Could you check a few things on this model? Use its own coordinates, in mm. Face numbers are marked on the shaded views. Round coordinates to 2 decimals unless told otherwise and drop trailing zeros. Loops run counter-clockwise (first coordinate to the right, second up) from the corner with the lowest first, then second, coordinate; pieces in that order, holes last. Notation, with made-up numbers: (2, 16) -> (6, 16) arc R35 cw to (6, 50) -> close; hole circle Ø3 at (16.25, -34.5). An arc over 180 degrees is marked (long way). Write each question's results on one line, items separated by ' | '. Start each with the question number.
1) Imagine slicing it at B-B, the plane y = 6.25. List the corners of the cut face in (x, z) for me (3 decimals), plus the area to 3 significant figures.
2) For P1, Ø4, axis at x = 47.5, z = -9, coming from the +Y side; P2, Ø1.5, axis at x = 37, y = 4.5, coming from the -Z side, each with a flat end and sliding along its axis, tell me the tip position at first contact or that it passes through.
3) Imagine slicing it at A-A, the plane z = -19.05. List the corners of the cut face in (x, y) for me (3 decimals).
4) If I drill on probe 1 along X at (y, z) = (1.05, -19.05) (3 decimals); probe 2 along X at (y, z) = (7.25, -5.5); probe 3 along X at (y, z) = (1.25, -20.5), over which ranges is the centre line in solid material (lowest first)?
5) Imagine slicing it at C-C, the plane x = 97.79. List the corners of the cut face in (y, z) for me (3 decimals).
6) We'd pull the mould along X, two halves only. Please class the marked faces 1 and 2: pulls with the +X half, pulls with the -X half, needs draft (parallel to the pull), parting line crosses it, or undercut.
7) Imagine slicing it at D-D, the plane z = -7.5. List the corners of the cut face in (x, y) for me, plus the area to 3 significant figures.
from build123d import *

# Parameters (mm, degrees)
BASE_R                 = 1.905
BOSS_EXTRUDEBASE_DEPTH = 2.54
STANDOFFS_R            = 3.175
STANDOFFS_R_2          = 1.27
BOSS_EXTRUDE2_DEPTH    = 5.08


with BuildPart() as part:
    # Base → Boss-ExtrudeBase (new body)
    with BuildSketch(Plane(origin=(0, 0, 0), x_dir=(1, 0, 0), z_dir=(0, 1, 0))):
        with BuildLine():
            Line((2.54, 0), (99.06, 0))
            ThreePointArc((99.06, 0), (100.856051224, 0.743948776), (101.6, 2.54))
            Line((101.6, 2.54), (101.6, 35.56))
            ThreePointArc((101.6, 35.56), (100.856051224, 37.356051224), (99.06, 38.1))
            Line((99.06, 38.1), (2.54, 38.1))
            ThreePointArc((2.54, 38.1), (0.743948776, 37.356051224), (0, 35.56))
            Line((0, 35.56), (0, 2.54))
            ThreePointArc((0, 2.54), (0.743948776, 0.743948776), (2.54, 0))
        make_face()
        with Locations(Location((3.81, 19.05, 0), (0, 0, 270))):
            Circle(BASE_R, mode=Mode.SUBTRACT)
        with Locations(Location((97.79, 19.05, 0), (0, 0, 90))):
            Circle(BASE_R, mode=Mode.SUBTRACT)
    extrude(amount=BOSS_EXTRUDEBASE_DEPTH)

    # Standoffs → Boss-Extrude2 (add)
    # profile 1 of 4: a face of its own
    with BuildSketch(Plane(origin=(0, 2.54, 0), x_dir=(1, 0, 0), z_dir=(0, 1, 0))):
        with Locations(Location((16.764, 32.766, 0), (0, 0, 90))):
            Circle(STANDOFFS_R)
        with Locations(Location((16.764, 32.766, 0), (0, 0, 270))):
            Circle(STANDOFFS_R_2, mode=Mode.SUBTRACT)
    # profile 2 of 4: a face of its own
    with BuildSketch(Plane(origin=(0, 2.54, 0), x_dir=(1, 0, 0), z_dir=(0, 1, 0))):
        with Locations(Location((84.836, 32.766, 0), (0, 0, 90))):
            Circle(STANDOFFS_R)
        with Locations(Location((84.836, 32.766, 0), (0, 0, 270))):
            Circle(STANDOFFS_R_2, mode=Mode.SUBTRACT)
    # profile 3 of 4: a face of its own
    with BuildSketch(Plane(origin=(0, 2.54, 0), x_dir=(1, 0, 0), z_dir=(0, 1, 0))):
        with Locations(Location((84.836, 5.334, 0), (0, 0, 90))):
            Circle(STANDOFFS_R)
        with Locations(Location((84.836, 5.334, 0), (0, 0, 270))):
            Circle(STANDOFFS_R_2, mode=Mode.SUBTRACT)
    # profile 4 of 4: a face of its own
    with BuildSketch(Plane(origin=(0, 2.54, 0), x_dir=(1, 0, 0), z_dir=(0, 1, 0))):
        with Locations(Location((16.764, 5.334, 0), (0, 0, 90))):
            Circle(STANDOFFS_R)
        with Locations(Location((16.764, 5.334, 0), (0, 0, 270))):
            Circle(STANDOFFS_R_2, mode=Mode.SUBTRACT)
    extrude(amount=BOSS_EXTRUDE2_DEPTH)


solid = part.part
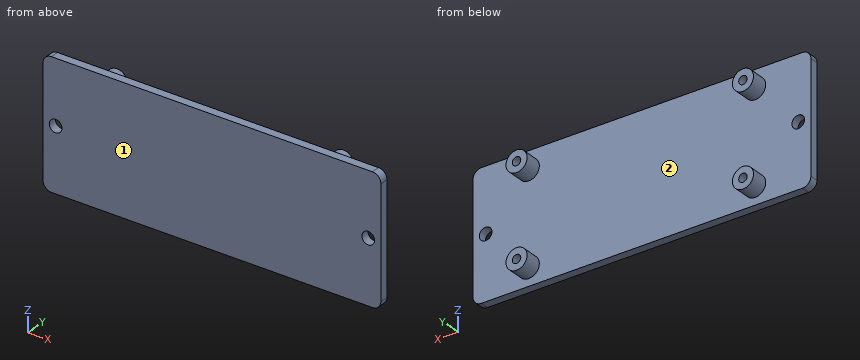
Checked values:
1) outline: circle Ø6.35 at (16.764, -32.766); circle Ø6.35 at (16.764, -5.334); circle Ø6.35 at (84.836, -32.766); circle Ø6.35 at (84.836, -5.334); hole circle Ø2.54 at (16.764, -32.766); hole circle Ø2.54 at (16.764, -5.334); hole circle Ø2.54 at (84.836, -32.766); hole circle Ø2.54 at (84.836, -5.334) | area: 106 mm^2
2) P1: y = 2.54 | P2: through
3) outline: (0, 0) -> (1.905, 0) -> (1.905, 2.54) -> (0, 2.54) -> close; (5.715, 0) -> (95.885, 0) -> (95.885, 2.54) -> (5.715, 2.54) -> close; (99.695, 0) -> (101.6, 0) -> (101.6, 2.54) -> (99.695, 2.54) -> close
4) probe 1: 0 to 1.905, 5.715 to 95.885, 99.695 to 101.6 | probe 2: 13.59 to 15.5, 18.02 to 19.93, 81.67 to 83.58, 86.1 to 88.01 | probe 3: 0 to 2.57, 5.05 to 96.55, 99.03 to 101.6
5) outline: (0, -38.1) -> (2.54, -38.1) -> (2.54, -20.955) -> (0, -20.955) -> close; (0, -17.145) -> (2.54, -17.145) -> (2.54, 0) -> (0, 0) -> close
6) face 1: needs draft | face 2: undercut
7) outline: (0, 0) -> (101.6, 0) -> (101.6, 2.54) -> (87.16, 2.54) -> (87.16, 7.62) -> (82.51, 7.62) -> (82.51, 2.54) -> (19.09, 2.54) -> (19.09, 7.62) -> (14.44, 7.62) -> (14.44, 2.54) -> (0, 2.54) -> close | area: 305 mm^2
